Here's the drawing with two shaded views (mm, measured from the low corner). I have some questions. A direction names the side the tool comes from. Coordinates: 2 decimals unless noted, no trailing zeros. Write each loop counter-clockwise with the first axis right and the second up, starting at its lowest first coordinate (ties: lowest second). Pieces come first, ordered by that corner, then holes. Notation, with made-up numbers: (22, 70.25) - (34, 70.25) arc R35 ccw to (34, 107.25) - close; hole circle Ø5 at (20.5, 65). An arc over 180 degrees is marked (long way). Answer in a Markdown table with one row per item. Add a question column.
Item 1: I'm going to push flat-ended pins straight in: pin 1 (1 mm diameter, centred on y = 45, z = 22, fed in from -X); pin 2 (5 mm diameter, centred on y = 28.5, z = 7.5, fed in from +X) (1 decimal); pin 3 (16 mm diameter, centred on x = 40, y = 40, fed in from -Z). Where does each tip first touch, or does it pass through?
Item 2: Imagine slicing it at A-A (y = 40). Please give me the cut outline in (x, z).
Item 3: If I drill on probe 1 along Y at (x, z) = (40, 12.75); probe 2 along Y at (x, z) = (41.5, 15.25); probe 3 along Z at (x, y) = (28.5, 48.5), over which ranges is the centre line in solid material (lowest first)? Write a range as from..to.
Item 4: Imagine slicing it at C-C (z = 26.25). Please give me the cut outline in (x, y).
Item 5: Imagine slicing it at D-D (y = 72). Please give me the cut outline in (x, z), plus the area to 3 significant figures.
Item 6: We'd pull the mould along X, two halves only. Please class the marked faces 1, 2, 3 and 4: +X half, -X half, draft (parallel to the pull), parting line (faces both ways), or undercut.
Item 7: Imagine slicing it at B-B (z = 12.75). Please give me the cut outline in (x, y), plus the area to 3 significant figures.
Item 8: Which directions (+Z, -Z, +X, -X, +Y, -Y) give clear straight access to the entire face, cutting with the end or side of a thin tool? Please do the marked faces 5 and 6.
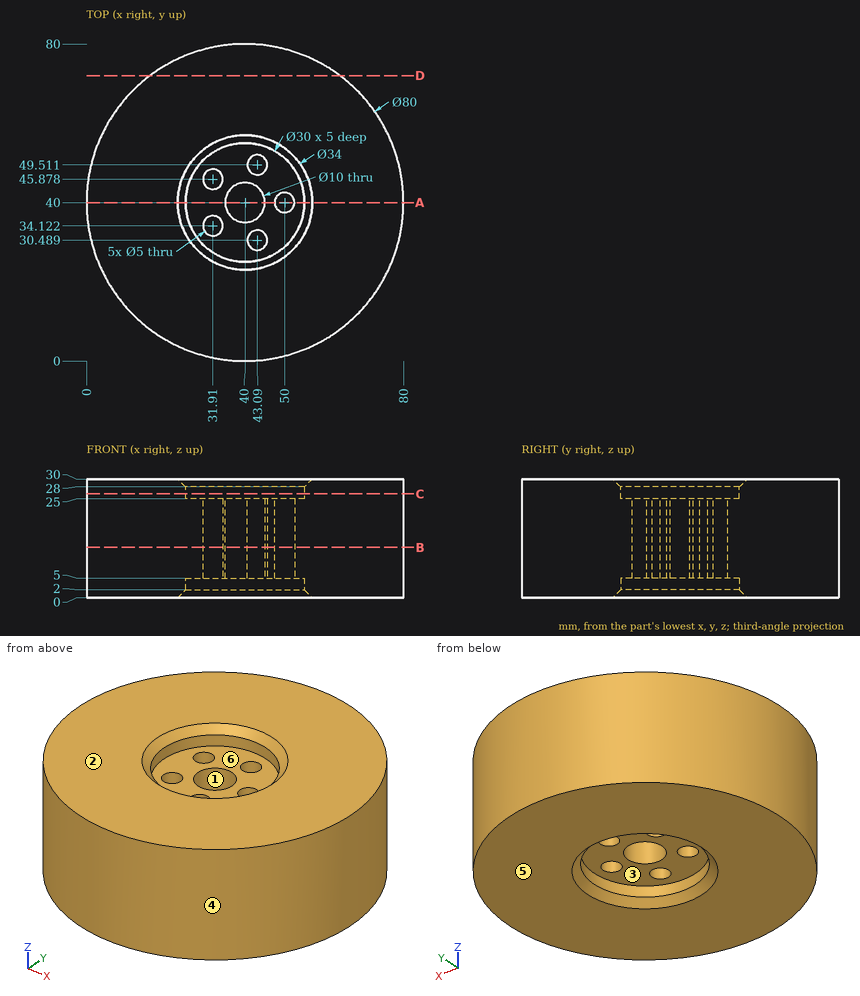
Here are the results:
| question | item | result |
|---|---|---|
| 1 | pin 1 | stops at x = 0.25 |
| 1 | pin 2 | stops at x = 79 |
| 1 | pin 3 | stops at z = 5 |
| 2 | outline | (0, 0) - (23, 0) - (25, 2) - (25, 5) - (35, 5) - (35, 25) - (25, 25) - (25, 28) - (23, 30) - (0, 30) - close; (45, 5) - (47.5, 5) - (47.5, 25) - (45, 25) - close; (52.5, 5) - (55, 5) - (55, 2) - (57, 0) - (80, 0) - (80, 30) - (57, 30) - (55, 28) - (55, 25) - (52.5, 25) - close |
| 3 | probe 1 | y = 0..35, 45..80 |
| 3 | probe 2 | y = 0.03..28.56, 32.42..35.23, 44.77..47.58, 51.44..79.97 |
| 3 | probe 3 | z = 5..25 |
| 4 | outline | circle Ø80 at (40, 40); hole circle Ø30 at (40, 40) |
| 5 | outline | (16, 0) - (64, 0) - (64, 30) - (16, 30) - close |
| 5 | area | 1,440 mm2 |
| 6 | face 1 | undercut |
| 6 | face 2 | draft |
| 6 | face 3 | undercut |
| 6 | face 4 | parting line |
| 7 | outline | circle Ø80 at (40, 40); hole circle Ø5 at (31.91, 34.12); hole circle Ø5 at (31.91, 45.88); hole circle Ø10 at (40, 40); hole circle Ø5 at (43.09, 30.49); hole circle Ø5 at (43.09, 49.51); hole circle Ø5 at (50, 40) |
| 7 | area | 4,850 mm2 |
| 8 | face 5 | -Z, +X, -X, +Y, -Y |
| 8 | face 6 | +Z |
